```python
from build123d import *

# Parameters (mm, degrees)
SKETCH1_W           = 36
SKETCH1_H           = 36
BOSS_EXTRUDE1_DEPTH = 4
CUT_EXTRUDE1_REACH  = 27.768
SKETCH2_R           = 2.75
BOSS_EXTRUDE2_DEPTH = 5
CHAMFER1_SIZE       = 4
SKETCH4_R           = 2.6
CUT_EXTRUDE2_DEPTH  = 7
BOSS_EXTRUDE3_DEPTH = 2.9


with BuildPart() as part:
    # Sketch1 → Boss-Extrude1 (new body)
    with BuildSketch(Plane.XY):
        Rectangle(SKETCH1_W, SKETCH1_H)
    extrude(amount=BOSS_EXTRUDE1_DEPTH)

    # Sketch2 → Cut-Extrude1 (cut, up to next)
    with BuildSketch(Plane.XY, mode=Mode.PRIVATE) as cut_extrude1_sk1:
        with Locations((-13, 13)):
            Circle(SKETCH2_R)
    cut_extrude1_tool1 = extrude(cut_extrude1_sk1.sketch, amount=CUT_EXTRUDE1_REACH, mode=Mode.PRIVATE) & part.part
    # Sketch2 → Cut-Extrude1 (cut, up to next)
    with BuildSketch(Plane.XY, mode=Mode.PRIVATE) as cut_extrude1_sk2:
        with Locations(Location((13, 13, 0), (0, 0, 180))):
            Circle(SKETCH2_R)
    cut_extrude1_tool2 = extrude(cut_extrude1_sk2.sketch, amount=CUT_EXTRUDE1_REACH, mode=Mode.PRIVATE) & part.part
    # Sketch2 → Cut-Extrude1 (cut, up to next)
    with BuildSketch(Plane.XY, mode=Mode.PRIVATE) as cut_extrude1_sk3:
        with Locations((13, -13)):
            Circle(SKETCH2_R)
    cut_extrude1_tool3 = extrude(cut_extrude1_sk3.sketch, amount=CUT_EXTRUDE1_REACH, mode=Mode.PRIVATE) & part.part
    # Sketch2 → Cut-Extrude1 (cut, up to next)
    with BuildSketch(Plane.XY, mode=Mode.PRIVATE) as cut_extrude1_sk4:
        with Locations(Location((-13, -13, 0), (0, 0, 180))):
            Circle(SKETCH2_R)
    cut_extrude1_tool4 = extrude(cut_extrude1_sk4.sketch, amount=CUT_EXTRUDE1_REACH, mode=Mode.PRIVATE) & part.part
    add(cut_extrude1_tool1.solids().sort_by_distance((-13, 13, 0))[0], mode=Mode.SUBTRACT)
    add(cut_extrude1_tool2.solids().sort_by_distance((13, 13, 0))[0], mode=Mode.SUBTRACT)
    add(cut_extrude1_tool3.solids().sort_by_distance((13, -13, 0))[0], mode=Mode.SUBTRACT)
    add(cut_extrude1_tool4.solids().sort_by_distance((-13, -13, 0))[0], mode=Mode.SUBTRACT)

    # Sketch3 → Boss-Extrude2 (add, symmetric)
    with BuildSketch(Plane(origin=(0, 0, 0), x_dir=(1, 0, 0), z_dir=(0, 1, 0))):
        with BuildLine():
            Line((-7, -4), (-7, -39))
            Line((-7, -39), (3, -39))
            Line((3, -39), (3, -31.849203781))
            ThreePointArc((3, -31.849203781), (-2.849203781, -22), (7, -16.150796219))
            Line((7, -16.150796219), (7, -4))
            Line((7, -4), (-7, -4))
        make_face()
    extrude(amount=BOSS_EXTRUDE2_DEPTH, both=True)

    # Chamfer1
    chamfer1_edges = [part.edges().sort_by_distance(p)[0] for p in [
        (0, -5, 4),
        (0, 5, 4),
    ]]
    chamfer(chamfer1_edges, length=CHAMFER1_SIZE)

    # Sketch4 → Cut-Extrude2 (cut, symmetric)
    with BuildSketch(Plane(origin=(0, 0, 0), x_dir=(0, 0, -1), z_dir=(1, 0, 0))):
        with Locations((-13, 0)):
            Circle(SKETCH4_R)
        with Locations((-35, 0)):
            Circle(SKETCH4_R)
    extrude(amount=CUT_EXTRUDE2_DEPTH, both=True, mode=Mode.SUBTRACT)

    # Sketch5 → Boss-Extrude3 (add, symmetric)
    with BuildSketch(Plane(origin=(0, 0, 0), x_dir=(1, 0, 0), z_dir=(0, 1, 0))):
        with BuildLine():
            Line((7, -15.738644179), (7, -18.343145751))
            ThreePointArc((7, -18.343145751), (-0.656854249, -22), (3, -29.656854249))
            Line((3, -29.656854249), (3, -32.261355821))
            ThreePointArc((3, -32.261355821), (-3.261355821, -22), (7, -15.738644179))
        make_face()
    extrude(amount=BOSS_EXTRUDE3_DEPTH, both=True)


solid = part.part
```
Could you check a few things on this model? Use its own coordinates, in mm. A direction names the side the tool comes from. Coordinates: 2 decimals unless noted, no trailing zeros. Order: outer loops, then holes, each group sorted by start corner. A loop starts at its lowest first (then second) coordinate and runs counter-clockwise, first axis right, second up. Notation, with made-up numbers: M 53,39 L 82,39 A22 ccw 82,64 Z; hole C -28,62.5 d4. An arc over 180 degrees is marked long. Use one line per item in the form item = value. Start each with the question number.
1. Suppose I cut it at D-D on y = -8. Write out the boundary of the cut face in (x, z), then the cut area to 3 significant figures.
2. Suppose I cut it at A-A on z = 35. Write out the boundary of the cut face in (x, y), then the cut area to 3 significant figures.
3. We'd pull the mould along X, two halves only. Please class faces 1 (the cylindrical face through (13.358, 10.273, 1.972)), 2 (the cylindrical face through (-1.9, 0.1, 37.6)), 3 (the flat face through (18, 0, 2)): +X half, -X half, draft (parallel to the pull), parting line (faces both ways), or undercut.
4. On a 3-axis mill with a long thin cutter (end or side, diameter ignored), from which of +Z, -Z, +X, -X, +Y, -Y can I reach the whole of each face in a straight line? I mean faces 4 (the cylindrical face through (5, 0, 15.5)), 5 (the flat face through (-7, 0, 21)), 6 (the flat face through (3, 0, 32)), 7 (the flat face through (-3, 5, 20)), 8 (the flat face through (-3, -5, 20)). Say none if no direction works.
5. Suppose I cut it at B-B on y = 0. Write out the boundary of the cut face in (x, z).
6. For pin 1 (3.5 mm diameter, centred on x = 13, y = -13, fed in from -Z); pin 2 (7 mm diameter, centred on y = 0, z = 8, fed in from +X); pin 3 (5.5 mm diameter, centred on y = -2, z = 17.5, fed in from -X); pin 4 (4.5 mm diameter, centred on y = -2, z = 35, fed in from +X), each with a flat end and sliding along its axis, tell me the tip position at first contact or that it passes through.
7. Suppose I cut it at C-C on x = 13. Write out the boundary of the cut face in (y, z), then the cut area to 3 significant figures.
8. Please list where these lines run through material, in increasing order: line 1 (Y direction, x = 13, z = 3.2); line 2 (Z direction, x = -4, y = 11.5).
Geometry says:
q1.outline = M -18,0 L 18,0 L 18,4 L 7,4 L 7,5 L -7,5 L -7,4 L -18,4 Z
q1.area = 158 mm^2
q2.outline = M -7,-5 L 3,-5 L 3,-2.6 L -7,-2.6 Z; M -7,2.6 L 3,2.6 L 3,5 L -7,5 Z
q2.area = 48.0 mm^2
q3.face_1 = undercut
q3.face_2 = draft
q3.face_3 = +X half
q4.face_4 = none
q4.face_5 = +Z, -X, +Y, -Y
q4.face_6 = +Z, +X, +Y, -Y
q4.face_7 = +Z, +X, -X, +Y
q4.face_8 = +Z, +X, -X, -Y
q5.outline = M -18,0 L 18,0 L 18,4 L 7,4 L 7,10.4 L -7,10.4 L -7,4 L -18,4 Z; M -7,15.6 L 3.7,15.6 A8.5 ccw 6.3,15.6 L 7,15.6 L 7,18.34 A6 cw 3,29.66 L 3,32.4 L -7,32.4 Z; M -7,37.6 L 3,37.6 L 3,39 L -7,39 Z
q6.pin_1 = through
q6.pin_2 = 7
q6.pin_3 = -7
q6.pin_4 = 3
q7.outline = M -18,0 L -15.75,0 L -15.75,4 L -18,4 Z; M -10.25,0 L 10.25,0 L 10.25,4 L -10.25,4 Z; M 15.75,0 L 18,0 L 18,4 L 15.75,4 Z
q7.area = 100 mm^2
q8.line_1 = -18 to -15.75, -10.25 to 10.25, 15.75 to 18
q8.line_2 = 0 to 4
